Source: CAD feature listing. Evaluate the final solid. Frame: model axes, mm. A direction names the side the tool comes from. Give positions to 0.01 mm unless a question says otherwise; leave off trailing zeros. Write each loop counter-clockwise with the first axis right and the second up, starting at its lowest first coordinate (ties: lowest second). Pieces come first, ordered by that corner, then holes.
```python
from build123d import *

# Parameters (mm, degrees)
SKETCH1_W           = 81.4
SKETCH1_H           = 6
BOSS_EXTRUDE1_DEPTH = 3
FILLET1_R           = 2
SKETCH2_R           = 1
BOSS_EXTRUDE2_DEPTH = 44
SKETCH3_W           = 81.4
SKETCH3_H           = 93
BOSS_EXTRUDE3_DEPTH = 2
FILLET2_R           = 2.5
SKETCH4_W           = 8
SKETCH4_H           = 4
BOSS_EXTRUDE4_DEPTH = 2


with BuildPart() as part:
    # Sketch1 → Boss-Extrude1 (new, symmetric)
    with BuildSketch(Plane(origin=(0, 0, 0), x_dir=(1, 0, 0), z_dir=(0, 1, 0))):
        Rectangle(SKETCH1_W, SKETCH1_H)
    extrude(amount=BOSS_EXTRUDE1_DEPTH, both=True)

    # Fillet1
    fillet1_edges = [part.edges().sort_by_distance(p)[0] for p in [
        (-40.7, 0, -3),
        (40.7, 0, -3),
        (40.7, 0, 3),
        (-40.7, 0, 3),
    ]]
    fillet(fillet1_edges, radius=FILLET1_R)

    # Sketch2 → Boss-Extrude2 (add, symmetric)
    with BuildSketch(Plane(origin=(0, 0, 0), x_dir=(0, 0, -1), z_dir=(1, 0, 0))):
        with Locations((0, 2)):
            Circle(SKETCH2_R)
    extrude(amount=BOSS_EXTRUDE2_DEPTH, both=True)

    # Sketch3 → Boss-Extrude3 (add)
    with BuildSketch(Plane.XZ.offset(3)):
        with Locations((0, 39.36)):
            Rectangle(SKETCH3_W, SKETCH3_H)
    extrude(amount=BOSS_EXTRUDE3_DEPTH)

    # Fillet2
    fillet2_edges = [part.edges().sort_by_distance(p)[0] for p in [
        (40.7, -4, -7.14),
        (40.7, -4, 85.86),
        (-40.7, -4, 85.86),
        (-40.7, -4, -7.14),
    ]]
    fillet(fillet2_edges, radius=FILLET2_R)

    # Sketch4 → Boss-Extrude4 (add)
    with BuildSketch(Plane.XZ.offset(5)):
        with Locations((0, 85.86)):
            Rectangle(SKETCH4_W, SKETCH4_H)
    extrude(amount=-BOSS_EXTRUDE4_DEPTH)


solid = part.part
```
1. Section query A-A (x = 2). Return loops of the section in (y, z), plus the area to 3 significant figures.
2. Pin query (flat end, axial travel): P1, Ø5, axis at x = -21.5, z = 75.5, coming from the +Y side; P2, Ø3, axis at y = -3.5, z = 3.5, coming from the -X side; P3, Ø1.5, axis at y = -2.5, z = 40, coming from the +X side. Return the tip coordinate at first contact, or that it passes through.
3. Line query: probe 1 along Y at (x, z) = (24.5, 59); probe 2 along Z at (x, y) = (-20, -3.25); probe 3 along Z at (x, y) = (12, -1). Output: solid intervals per line, ascending.
4. Access query for faces 1 (the cylindrical face through (-40.13, -0.04, -2.4)), 2 (the flat face through (-1, 0, 3)), 3 (the cylindrical face through (-42, 1, 0)), 4 (the cylindrical face through (-40.13, 0.04, 2.4)), 5 (the flat face through (4, -4, 87)). Directions: +Z, -Z, +X, -X, +Y, -Y. A direction counts if a zero-diameter tool reaches every point of the face in a straight line with its end or side. Return the directions, or none.
5. Section query B-B (z = 66). Return loops of the section in (x, y).
The answers:
1. outline: (-5, -7.14) - (-3, -7.14) - (-3, -3) - (3, -3) - (3, 3) - (-3, 3) - (-3, 87.86) - (-5, 87.86) - close
1. area: 226 mm2
2. P1: stops at y = -3
2. P2: stops at x = -40.7
2. P3: stops at x = 40.7
3. probe 1: y = -5 to -3
3. probe 2: z = -7.14 to 85.86
3. probe 3: z = -3 to 3
4. face 1: -Z, -X, +Y
4. face 2: +Z, +X, -X, +Y
4. face 3: -X
4. face 4: +Z, -X, +Y
4. face 5: +Z, +X, +Y, -Y
5. outline: (-40.7, -5) - (40.7, -5) - (40.7, -3) - (-40.7, -3) - close
